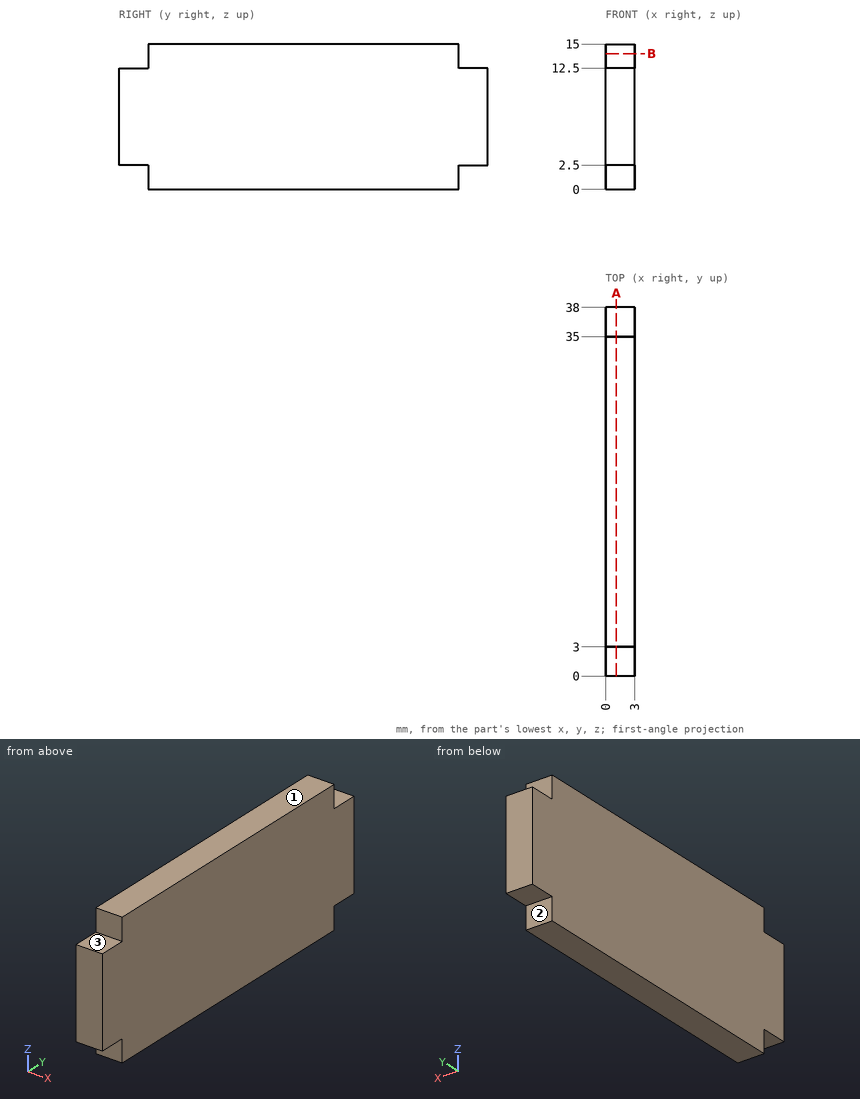
Source: three-view drawing plus pictorial views. Frame: mm from the lowest corner of the part. A direction names the side the tool comes from. Round coordinates to 2 decimals unless told otherwise and drop trailing zeros. Loops run counter-clockwise (first coordinate to the right, second up) from the corner with the lowest first, then second, coordinate; pieces in that order, holes last.
1. Section query B-B on z = 14. Output: boundary loops of the cut face in (x, y).
2. Section query A-A on x = 1.1. Output: boundary loops of the cut face in (y, z).
3. Ray query, L1, parallel to Y at x = 2.65, z = 2; L2, parallel to Z at x = 0.55, y = 36. Return the intervals inside material, ascending.
4. Access query for the marked faces 1, 2 and 3. Directions: +Z, -Z, +X, -X, +Y, -Y. A direction counts if a zero-diameter tool reaches every point of the face in a straight line with its end or side. Return the directions, or none.
5. Contact query for flat-ended pins moving along their axis: pin 1 (0.8 mm diameter, centred on x = 1.5, z = 13.5, fed in from -Y); pin 2 (1.5 mm diameter, centred on x = 1.5, y = 2, fed in from -Z); pin 3 (1.2 mm diameter, centred on x = 1.5, z = 14, fed in from +Y). Output: stop coordinate, or through.
Answers below:
1. outline: (0, 3) - (3, 3) - (3, 35) - (0, 35) - close
2. outline: (0, 2.5) - (3, 2.5) - (3, 0) - (35, 0) - (35, 2.5) - (38, 2.5) - (38, 12.5) - (35, 12.5) - (35, 15) - (3, 15) - (3, 12.5) - (0, 12.5) - close
3. L1: y = 3 to 35
3. L2: z = 2.5 to 12.5
4. face 1: +Z, +X, -X, +Y, -Y
4. face 2: -Z, +X, -X, +Y
4. face 3: +Z, +X, -X, -Y
5. pin 1: stops at y = 3
5. pin 2: stops at z = 2.5
5. pin 3: stops at y = 35
